```python
from build123d import *

# Parameters (mm, degrees)
SKETCH2_R           = 2.778125
BOSS_EXTRUDE2_DEPTH = 56.3835756
SKETCH3_R           = 1.651
CUT_EXTRUDE1_DEPTH  = 22.1668
SKETCH4_W           = 10.767766953
SKETCH4_H           = 2.34
CUT_EXTRUDE2_DEPTH  = 3.75
SKETCH5_R           = 2.8
CUT_EXTRUDE3_DEPTH  = 80.995318373
SKETCH6_R           = 1.905
CUT_EXTRUDE4_DEPTH  = 77.107177875
CUT_EXTRUDE5_DEPTH  = 4


with BuildPart() as part:
    # Sketch2 → Boss-Extrude2 (new body)
    with BuildSketch(Plane(origin=(0, 0, 0), x_dir=(0, 0, -1), z_dir=(1, 0, 0))):
        with BuildLine():
            Line((0, 25.778125), (30, 25.778125))
            ThreePointArc((30, 25.778125), (31.964431026, 24.964431026), (32.778125, 23))
            Line((32.778125, 23), (32.778125, 14.278125))
            ThreePointArc((32.778125, 14.278125), (31.964431026, 12.313693974), (30, 11.5))
            Line((30, 11.5), (30, 6.906829453))
            Line((30, 6.906829453), (31.767766953, 5.1390625))
            Line((31.767766953, 5.1390625), (46.767766953, 5.1390625))
            Line((46.767766953, 5.1390625), (46.767766953, 32.1390625))
            Line((46.767766953, 32.1390625), (-16.767766953, 32.1390625))
            Line((-16.767766953, 32.1390625), (-16.767766953, 5.1390625))
            Line((-16.767766953, 5.1390625), (-1.767766953, 5.1390625))
            Line((-1.767766953, 5.1390625), (0, 6.906829453))
            Line((0, 6.906829453), (0, 11.5))
            ThreePointArc((0, 11.5), (-1.964431026, 12.313693974), (-2.778125, 14.278125))
            Line((-2.778125, 14.278125), (-2.778125, 23))
            ThreePointArc((-2.778125, 23), (-1.964431026, 24.964431026), (0, 25.778125))
        make_face()
        with Locations((-10, 26.6390625)):
            Circle(SKETCH2_R, mode=Mode.SUBTRACT)
        with Locations((-10, 10.6390625)):
            Circle(SKETCH2_R, mode=Mode.SUBTRACT)
        with Locations(Location((40, 10.6390625, 0), (0, 0, 180))):
            Circle(SKETCH2_R, mode=Mode.SUBTRACT)
        with Locations(Location((40, 26.6390625, 0), (0, 0, 180))):
            Circle(SKETCH2_R, mode=Mode.SUBTRACT)
    extrude(amount=BOSS_EXTRUDE2_DEPTH)

    # Sketch3 → Cut-Extrude1 (cut)
    with BuildSketch(Plane(origin=(56.3835756, 0, 0), x_dir=(0, 0, -1), z_dir=(1, 0, 0))):
        with Locations((-10, 18.6390625)):
            Circle(SKETCH3_R)
        with Locations(Location((40, 18.6390625, 0), (0, 0, 180))):
            Circle(SKETCH3_R)
    cut_extrude1 = extrude(amount=-CUT_EXTRUDE1_DEPTH, mode=Mode.SUBTRACT)

    # Sketch4 → Cut-Extrude2 (cut, symmetric)
    with BuildSketch(Plane(origin=(0, 18.6390625, 0), x_dir=(0, 0, -1), z_dir=(0, -1, 0))):
        with Locations((-11.383883477, 45.2135756)):
            Rectangle(SKETCH4_W, SKETCH4_H)
        with Locations((41.383883477, 45.2135756)):
            Rectangle(SKETCH4_W, SKETCH4_H)
        with Locations((-11.383883477, 8.83)):
            Rectangle(SKETCH4_W, SKETCH4_H)
        with Locations((41.383883477, 8.83)):
            Rectangle(SKETCH4_W, SKETCH4_H)
    extrude(amount=CUT_EXTRUDE2_DEPTH, both=True, mode=Mode.SUBTRACT)

    # Sketch5 → Cut-Extrude3 (cut, through all)
    with BuildSketch(Plane(origin=(56.3835756, 0, 0), x_dir=(0, 0, -1), z_dir=(1, 0, 0))):
        with Locations((-10, 26.6390625)):
            Circle(SKETCH5_R)
        with Locations((0, 23)):
            Circle(SKETCH5_R)
        with Locations((-10, 10.6390625)):
            Circle(SKETCH5_R)
        with Locations((40, 26.6390625)):
            Circle(SKETCH5_R)
        with Locations((40, 10.6390625)):
            Circle(SKETCH5_R)
        with Locations((30, 23)):
            Circle(SKETCH5_R)
        with Locations((0, 14.278125)):
            Circle(SKETCH5_R)
        with Locations((30, 14.278125)):
            Circle(SKETCH5_R)
    extrude(amount=-CUT_EXTRUDE3_DEPTH, mode=Mode.SUBTRACT)

    # Mirror1: Cut-Extrude1 across plane
    add(cut_extrude1.mirror(Plane.ZY.offset(-28.1917878)), mode=Mode.SUBTRACT)

    # Sketch6 → Cut-Extrude4 (cut, through all)
    with BuildSketch(Plane.XZ.offset(-25.778125)):
        with Locations(Location((8.949145412, -5, 0), (0, 0, 270))):
            Circle(SKETCH6_R)
        with Locations(Location((47.434430188, -5, 0), (0, 0, 270))):
            Circle(SKETCH6_R)
        with Locations(Location((47.434430188, -25, 0), (0, 0, 270))):
            Circle(SKETCH6_R)
        with Locations(Location((8.949145412, -25, 0), (0, 0, 270))):
            Circle(SKETCH6_R)
    extrude(amount=-CUT_EXTRUDE4_DEPTH, mode=Mode.SUBTRACT)

    # Sketch7 → Cut-Extrude5 (cut)
    with BuildSketch(Plane(origin=(0, 25.778125, 0), x_dir=(-1, 0, 0), z_dir=(0, -1, 0))):
        Polygon((-12.166931132, 27.281957343), (-12.534271302, 23.354294494), (-9.316485582, 21.072337151), (-5.731359693, 22.718042657), (-5.364019523, 26.645705506), (-8.581805243, 28.927662849), align=None)
        Polygon((-12.465792586, 6.787363117), (-12.255370864, 2.84817577), (-8.73872369, 1.060812653), (-5.432498239, 3.212636883), (-5.642919961, 7.15182423), (-9.159567134, 8.939187347), align=None)
        Polygon((-44.671186116, 7.815307524), (-48.490935987, 8.800693325), (-51.254180059, 5.985385801), (-50.197674259, 2.184692476), (-46.377924389, 1.199306675), (-43.614680317, 4.014614199), align=None)
        Polygon((-43.896441738, 26.74473837), (-47.176423714, 28.936357061), (-50.714412164, 27.191618691), (-50.972418638, 23.25526163), (-47.692436661, 21.063642939), (-44.154448211, 22.808381309), align=None)
    extrude(amount=-CUT_EXTRUDE5_DEPTH, mode=Mode.SUBTRACT)


solid = part.part
```
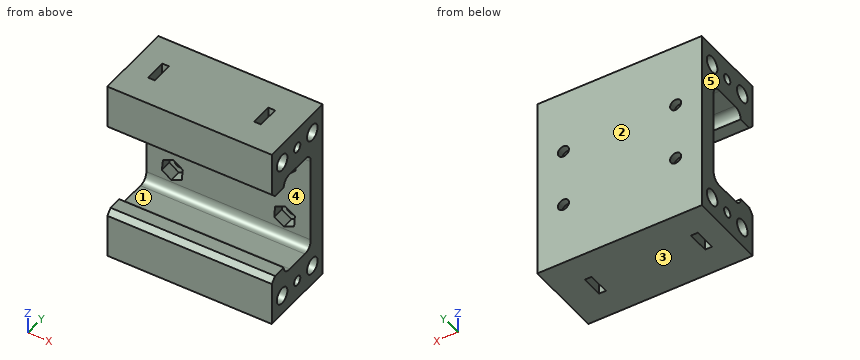
Source: CAD feature listing. Evaluate the final solid. Frame: model axes, mm. Face numbers are marked on the shaded views. A direction names the side the tool comes from. Coordinates: 2 decimals unless noted, no trailing zeros. Loops run counter-clockwise (first coordinate to the right, second up) from the corner with the lowest first, then second, coordinate; pieces in that order, holes last. Notation, with made-up numbers: (43, -14) - (86, -14) arc R19 ccw to (86, -5) - close; hole circle Ø4 at (-13, 61.5). An arc over 180 degrees is marked (long way). Answer as CSV lines item,"result".
1. Reachability of the marked faces 1 and 2 from +Z, -Z, +X, -X, +Y, -Y: full face, straight path, thin tool, end or side. Return the list, or none.
Established:
face 1,"+X, -X"
face 2,"+Z, -Z, +X, -X, +Y"
2. Section D-D (x = 16). Return loops of the section in (y, z), then the cut area to 3 significant figures.
Established:
outline,"(5.14, -46.77) - (32.14, -46.77) - (32.14, 16.77) - (5.14, 16.77) - (5.14, 1.77) - (6.91, 0) - (11.48, 0) arc R2.8 cw to (14.63, 2.78) - (22.65, 2.78) arc R2.8 cw to (25.78, -0.35) - (25.78, -29.65) arc R2.8 cw to (22.65, -32.78) - (14.63, -32.78) arc R2.8 cw to (11.48, -30) - (6.91, -30) - (5.14, -31.77) - close; hole circle Ø5.6 at (10.64, -40); hole circle Ø5.6 at (10.64, 10); hole circle Ø3.3 at (18.64, -40); hole circle Ø3.3 at (18.64, 10); hole circle Ø5.6 at (26.64, -40); hole circle Ø5.6 at (26.64, 10)"
area,"904 mm2"
3. Section A-A (y = 16.25). Return loops of the section in (x, z).
Established:
outline,"(0, -46.77) - (7.66, -46.77) - (7.66, -36) - (10, -36) - (10, -46.77) - (44.04, -46.77) - (44.04, -36) - (46.38, -36) - (46.38, -46.77) - (56.38, -46.77) - (56.38, -32.78) - (0, -32.78) - close; (0, 2.78) - (56.38, 2.78) - (56.38, 16.77) - (46.38, 16.77) - (46.38, 6) - (44.04, 6) - (44.04, 16.77) - (10, 16.77) - (10, 6) - (7.66, 6) - (7.66, 16.77) - (0, 16.77) - close"
4. Ray query, line 1 (Y direction, x = 29, z = -40); line 2 (Y direction, x = 51, z = 10); line 3 (Z direction, x = 21, y = 23). Return the intervals inside material, ascending.
Established:
line 1,"y = 5.14 to 7.84, 13.44 to 23.84, 29.44 to 32.14"
line 2,"y = 5.14 to 7.84, 13.44 to 16.99, 20.29 to 23.84, 29.44 to 32.14"
line 3,"z = -46.77 to -32.8, 2.8 to 16.77"
5. Section C-C (y = 12.5). Return loops of the section in (x, z).
Established:
outline,"(0, -46.77) - (56.38, -46.77) - (56.38, -42.09) - (0, -42.09) - close; (0, -37.91) - (56.38, -37.91) - (56.38, -32.16) - (0, -32.16) - close; (0, 2.16) - (56.38, 2.16) - (56.38, 7.91) - (0, 7.91) - close; (0, 12.09) - (56.38, 12.09) - (56.38, 16.77) - (0, 16.77) - close"
6. Section B-B (z = -5). Return loops of the section in (x, y), then the cut area to 3 significant figures.
Established:
outline,"(0, 25.78) - (5.53, 25.78) - (5.53, 29.78) - (7.04, 29.78) - (7.04, 32.14) - (0, 32.14) - close; (10.85, 29.78) - (12.37, 29.78) - (12.37, 25.78) - (43.89, 25.78) - (43.89, 29.78) - (45.53, 29.78) - (45.53, 32.14) - (10.85, 32.14) - close; (49.34, 29.78) - (50.98, 29.78) - (50.98, 25.78) - (56.38, 25.78) - (56.38, 32.14) - (49.34, 32.14) - close"
area,"285 mm2"
7. Mould query, pull axis Z, two halves, no side actions, for the marked faces 3, 4 and 5. Classes: released by +Z, released by -Z, zero draft, split by the parting line, or undercut.
Established:
face 3,"released by -Z"
face 4,"undercut"
face 5,"zero draft"
8. Contact query for flat-ended pins moving along their axis: pin 1 (3 mm diameter, centred on x = 8.95, z = -5, fed in from +Y); pin 2 (3.5 mm diameter, centred on x = 7.5, z = -25.5, fed in from -Y); pin 3 (9 mm diameter, centred on x = 24, z = -22, fed in from -Y). Output: stop coordinate, or through.
Established:
pin 1,"passes through"
pin 2,"stops at y = 29.78"
pin 3,"stops at y = 25.78"
